Autodesk Inventor part; units mm, degrees
ref_plane "YZ Plane" through (0, 0, 0) normal (1, 0, 0) x (0, 1, 0)
ref_plane "XZ Plane" through (0, 0, 0) normal (0, 1, 0) x (-1, 0, 0)
ref_plane "XY Plane" through (0, 0, 0) normal (0, 0, 1) x (1, 0, 0)
sketch "Sketch1" plane through (0, 0, 0) normal (0, 1, 0) x (-1, 0, 0)
  circle A0 centre (0, 0) radius 3.25
  circle A1 centre (0, 0) radius 6
  dimension "d0" = 6.5
  dimension "d1" = 12
extrude "Extrusion1" add sketch "Sketch1" along normal blind 13.5
sketch "Sketch2" plane through (0, 13.5, 0) normal (0, 1, 0) x (1, 0, 0)
  line L0 (0, 0) -> (25, 0) construction
  line L1 (25, 7.5) -> (40, 7.5) construction
  line L2 (40, 7.5) -> (40, -7.5) construction
  line L3 (40, -7.5) -> (25, -7.5) construction
  line L4 (25, -7.5) -> (25, 7.5) construction
  circle A0 centre (25, 7.5) radius 1.4
  circle A1 centre (40, 7.5) radius 1.4
  circle A2 centre (40, -7.5) radius 1.4
  circle A3 centre (25, -7.5) radius 1.4
  circle A4 centre (0, 0) radius 6.3 construction
  line L5 (40.5, 11.5) -> (21, 11.5)
  line L6 (21, -11.5) -> (40.5, -11.5)
  line L7 (44, -8) -> (44, 8)
  line L8 (21, 11.5) -> (-1.4711, 5.8169)
  line L9 (21, -11.5) -> (-1.4711, -5.8169)
  circle A5 centre (0, 0) radius 6
  circle A6 centre (0, 0) radius 3.25
  arc A7 (44, 8) -> (40.5, 11.5) centre (40.5, 8) ccw
  arc A8 (40.5, -11.5) -> (44, -8) centre (40.5, -8) ccw
  dimension "d4" = 25
  dimension "d5" = 15
  dimension "d6" = 15
  dimension "d7" = 7.5
  dimension "d8" = 2.8
  dimension "d9" = 2.8
  dimension "d10" = 2.8
  dimension "d11" = 2.8
  dimension "d12" = 12.6
  dimension "d13" = 4
  dimension "d14" = 3.5
extrude "Extrusion2" add sketch "Sketch2" along normal blind 3
fillet "Fillet1" radius 0.8 4 edges at (23.6, 16.5, 7.5) (23.6, 16.5, -7.5) (38.6, 16.5, -7.5) (38.6, 16.5, 7.5)
sketch "Sketch3" plane through (0, 13.5, 0) normal (0, -1, 0) x (1, 0, 0)
  circle A0 centre (0, 0) radius 6
  line L0 (5.9161, 1) -> (16, 1)
  line L1 (5.9161, -1) -> (16, -1)
  line L2 (16, 1) -> (16, -1)
  dimension "d18" = 1
  dimension "d19" = 1
  dimension "d20" = 10
extrude "Extrusion3" add sketch "Sketch3" along normal blind 10 contours A0 L0 L2 L1
chamfer "Chamfer1" distance 10 angle 45 1 edges at (16, 3.5, 0)
equation "\"d7\" = 0.5 * d6"
equation "\"d9\" = d8"
equation "\"d10\" = d8"
equation "\"d11\" = d8"
properties part number "WM 720p USB Webcam Endefector Mount"
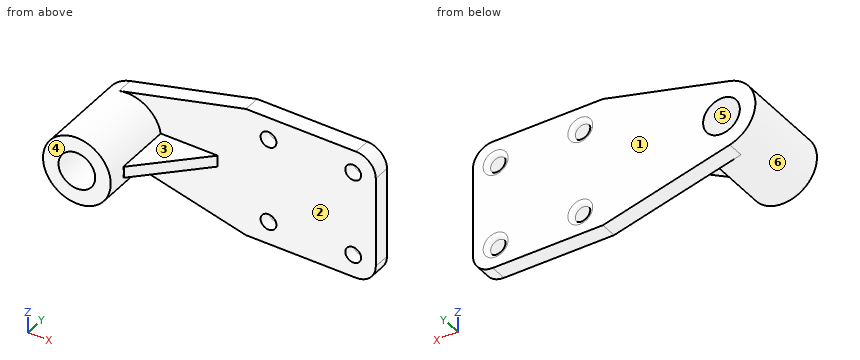
Read the model definition and answer for the solid it produces. Units are mm, in the model's axes. Face numbers are marked on the shaded views. A direction names the side the tool comes from. Give positions to 0.01 mm unless a question says otherwise; leave off trailing zeros. Write each loop counter-clockwise with the first axis right and the second up, starting at its lowest first coordinate (ties: lowest second). Pieces come first, ordered by that corner, then holes. Notation, with made-up numbers: (4, 57.25) -> (48, 57.25) arc R19 ccw to (48, 73.25) -> close; hole circle Ø9 at (61.25, 53). An arc over 180 degrees is marked (long way). Answer in a Markdown table with one row per item.
1) Each of these flat-tipped pins is pushed along its axis until it touches: pin 1 Ø3 at (x, y) = (9.5, 7.5) entering from -Z; pin 2 Ø1.5 at (x, z) = (28, 4.5) entering from -Y. Where does it stop, or does it pass through?
Results list:
| item | result |
|---|---|
| pin 1 | z = -1 |
| pin 2 | y = 13.5 |
2) Section B-B on z = 7.5 is taken. Give the vertices of the cut face in (x, y).
Results list:
| item | result |
|---|---|
| outline | (5.18, 13.5) -> (23.6, 13.5) -> (23.6, 15.7) arc R0.8 ccw to (22.8, 16.5) -> (5.18, 16.5) -> close; (26.4, 13.5) -> (38.6, 13.5) -> (38.6, 15.7) arc R0.8 ccw to (37.8, 16.5) -> (27.2, 16.5) arc R0.8 ccw to (26.4, 15.7) -> close; (41.4, 13.5) -> (44, 13.5) -> (44, 16.5) -> (42.2, 16.5) arc R0.8 ccw to (41.4, 15.7) -> close |
3) Section D-D on y = 10.25 is taken. Give the vertices of the cut face in (x, z), plus the area to 3 significant figures.
Results list:
| item | result |
|---|---|
| outline | (5.92, -1) -> (12.75, -1) -> (12.75, 1) -> (5.92, 1) arc R6 ccw (long way) to start; hole circle Ø6.5 at (0, 0) |
| area | 93.5 mm^2 |
4) Section A-A on x = 25 is taken. Give the vertices of the cut face in (y, z), plus the area to 3 significant figures.
Results list:
| item | result |
|---|---|
| outline | (13.5, -11.5) -> (16.5, -11.5) -> (16.5, -9.7) arc R0.8 ccw to (15.7, -8.9) -> (13.5, -8.9) -> close; (13.5, -6.1) -> (15.7, -6.1) arc R0.8 ccw to (16.5, -5.3) -> (16.5, 5.3) arc R0.8 ccw to (15.7, 6.1) -> (13.5, 6.1) -> close; (13.5, 8.9) -> (15.7, 8.9) arc R0.8 ccw to (16.5, 9.7) -> (16.5, 11.5) -> (13.5, 11.5) -> close |
| area | 51.7 mm^2 |
5) A tool of negligible diameter and unlimited length cuts with its end or side. For the marked faces 1, 2 and 3, from which of +Z, -Z, +X, -X, +Y, -Y can it reach the whole face along a straight path? Write none if from no direction.
Results list:
| item | result |
|---|---|
| face 1 | +Z, -Z, +X, -X, +Y |
| face 2 | +X, -Y |
| face 3 | +Z, +X, -Y |
6) Determine the mould class of the marked faces 4, 5 and 6 for opening direction X: released by +X, released by -X, zero draft, split by the parting line, or undercut.
Results list:
| item | result |
|---|---|
| face 4 | zero draft |
| face 5 | undercut |
| face 6 | split by the parting line |
7) Section C-C on z = -2.25 is taken. Give the vertices of the cut face in (x, y), plus the area to 3 significant figures.
Results list:
| item | result |
|---|---|
| outline | (-5.56, 0) -> (-2.35, 0) -> (-2.35, 16.5) -> (-5.56, 16.5) -> close; (2.35, 0) -> (5.56, 0) -> (5.56, 13.5) -> (44, 13.5) -> (44, 16.5) -> (2.35, 16.5) -> close |
| area | 221 mm^2 |
8) Straight lines are drawn through the part: line 1 (Z direction, x = 25, y = 14); line 2 (Z direction, x = 41, y = 15); line 3 (Y direction, x = 6, z = 4.25). For each, find the intervals that lie inside material, in ascending order. Write a range as [from, to].
Results list:
| item | result |
|---|---|
| line 1 | [-11.5, -8.9], [-6.1, 6.1], [8.9, 11.5] |
| line 2 | [-11.46, -8.48], [-6.52, 6.52], [8.48, 11.46] |
| line 3 | [13.5, 16.5] |
